Work out the finished part from the listing and answer in its coordinate system (mm). Face numbers are marked on the shaded views. Coordinates: 2 decimals unless noted, no trailing zeros. Order: outer loops, then holes, each group sorted by start corner. A loop starts at its lowest first (then second) coordinate and runs counter-clockwise, first axis right, second up. Notation, with made-up numbers: (17, 45.25) -> (27, 45.25) arc R28 ccw to (27, 79.25) -> close; hole circle Ø1 at (77.25, 37.25). An arc over 180 degrees is marked (long way). Answer as CSV lines item,"result". Start each with the question number.
Item 1: Each of these flat-tipped pins is pushed along its axis until it touches: pin 1 Ø11 at (x, z) = (87.5, -304.5) entering from +Y; pin 2 Ø1 at (x, z) = (195, -235.5) entering from +Y; pin 3 Ø5 at (x, z) = (173, -341.5) entering from +Y. Where does it stop, or does it pass through?
Item 2: For a pull along Z with two mould halves and no side action, classify the marked faces 1 and 2 as pulls with the +Z half, pulls with the -Z half, needs draft (parallel to the pull), parting line crosses it, or undercut.
Item 3: Section A-A (x = 214) is taken. Write down the section's boundary in (y, z), then the cut area to 3 significant figures.
Item 4: Straight lines are drawn through the part: L1, parallel to X at y = 12.25, z = -313; L2, parallel to X at y = 3.25, z = -337.5; L3, parallel to Z at x = 127, y = 2.75. For each, find the intervals that lie inside material, in ascending order.
```python
from build123d import *

# Parameters (mm, degrees)
SKETCH1_W                     = 224.81
SKETCH1_H                     = 138.7
BOTTOM_PLATE_DEPTH            = 4
SKETCH2_W                     = 8
SKETCH2_H                     = 8
SKETCH2_W_2                   = 7
SKETCH2_H_2                   = 7
SIDE_WALLS_DEPTH              = 11
SKETCH11_W                    = 4
SKETCH11_H                    = 123.7
USB_CUTOUT_DEPTH              = 11
CSK_FOR_M3_SFHCS1_D           = 3.2
CSK_FOR_M3_SFHCS1_CSINK_D     = 6.72
CSK_FOR_M3_SFHCS1_CSINK_ANGLE = 90
FILLET1_R                     = 1.5
USB_C_PORT_DEPTH              = 10
SKETCH18_W                    = 15
SKETCH18_H                    = 4.1
BOSS_EXTRUDE1_DEPTH           = 1.5
CHAMFER1_SIZE                 = 2
SKETCH16_R                    = 5
PCB_SUPPORT_DEPTH             = 2
SKETCH17_R                    = 1.5
ALIGNMENT_POSTS_DEPTH         = 2
SKETCH20_R                    = 1.6
PCB_SCREW_CLEARANCE_DEPTH     = 2.15
SKETCH21_W                    = 5.5
SKETCH21_H                    = 5.5
CUT_EXTRUDE2_DEPTH            = 1.8


with BuildPart() as part:
    # Sketch1 → bottom_plate (new body)
    with BuildSketch(Plane(origin=(0, 0, 0), x_dir=(1, 0, 0), z_dir=(0, 1, 0))):
        with Locations((157.396993286, 282.353126042)):
            Rectangle(SKETCH1_W, SKETCH1_H)
    extrude(amount=BOTTOM_PLATE_DEPTH)

    # Sketch2 → side_walls (add)
    with BuildSketch(Plane(origin=(0, 4, 0), x_dir=(1, 0, 0), z_dir=(0, 1, 0))):
        with Locations((48.991993286, 217.003126042)):
            Rectangle(SKETCH2_W, SKETCH2_H)
        with Locations((266.301993286, 216.503126042)):
            Rectangle(SKETCH2_W_2, SKETCH2_H_2)
        with Locations((266.301993286, 348.203126042)):
            Rectangle(SKETCH2_W_2, SKETCH2_H_2)
        with Locations((48.991993286, 348.203126042)):
            Rectangle(SKETCH2_W, SKETCH2_H_2)
    extrude(amount=SIDE_WALLS_DEPTH)

    # Sketch11 → usb_cutout (add)
    with BuildSketch(Plane(origin=(0, 4, 0), x_dir=(1, 0, 0), z_dir=(0, 1, 0))):
        with Locations((46.991993286, 282.853126042)):
            Rectangle(SKETCH11_W, SKETCH11_H)
        Polygon((52.991993286, 213.003126042), (262.801993286, 213.003126042), (262.801993286, 219.003126042), (269.801993286, 219.003126042), (269.801993286, 345.703126042), (262.801993286, 345.703126042), (262.801993286, 351.703126042), (52.991993286, 351.703126042), (52.991993286, 345.703126042), (75.991993286, 345.703126042), (75.991993286, 349.803126042), (90.991993286, 349.803126042), (90.991993286, 345.703126042), (261.801993286, 345.703126042), (261.801993286, 219.003126042), (52.991993286, 219.003126042), align=None)
    extrude(amount=USB_CUTOUT_DEPTH)

    # CSK for M3 SFHCS1 (through all)
    with Locations(Plane(origin=(0, 0, 0), x_dir=(-1, 0, 0), z_dir=(0, -1, 0))):
        with Locations((-48.991993286, 217.003686618), (-265.799879733, 217.003686618), (-265.799879733, 347.703126042), (-48.991993286, 347.703126042)):
            CounterSinkHole(CSK_FOR_M3_SFHCS1_D / 2, CSK_FOR_M3_SFHCS1_CSINK_D / 2, counter_sink_angle=CSK_FOR_M3_SFHCS1_CSINK_ANGLE)

    # Fillet1
    fillet1_edges = [part.edges().sort_by_distance(p)[0] for p in [
        (44.991993286, 7.5, -351.703126042),
        (269.801993286, 7.5, -351.703126042),
        (269.801993286, 7.5, -213.003126042),
        (44.991993286, 7.5, -213.003126042),
    ]]
    fillet(fillet1_edges, radius=FILLET1_R)

    # Sketch14 → usb-c port (cut)
    with BuildSketch(Plane.XY.offset(-349.803126042)):
        with BuildLine():
            Line((80.300245901, 7.7), (86.470717131, 7.7))
            ThreePointArc((86.470717131, 7.7), (87.531377303, 8.139339828), (87.970717131, 9.2))
            Line((87.970717131, 9.2), (87.970717131, 9.590467347))
            ThreePointArc((87.970717131, 9.590467347), (87.531377303, 10.651127519), (86.470717131, 11.090467347))
            Line((86.470717131, 11.090467347), (80.300245901, 11.090467347))
            ThreePointArc((80.300245901, 11.090467347), (79.239585729, 10.651127519), (78.800245901, 9.590467347))
            Line((78.800245901, 9.590467347), (78.800245901, 9.2))
            ThreePointArc((78.800245901, 9.2), (79.239585729, 8.139339828), (80.300245901, 7.7))
        make_face()
    extrude(amount=-USB_C_PORT_DEPTH, mode=Mode.SUBTRACT)

    # Sketch18 → Boss-Extrude1 (add)
    with BuildSketch(Plane(origin=(0, 15, 0), x_dir=(1, 0, 0), z_dir=(0, 1, 0))):
        with Locations((83.491993286, 347.753126042)):
            Rectangle(SKETCH18_W, SKETCH18_H)
    extrude(amount=-BOSS_EXTRUDE1_DEPTH)

    # Chamfer1
    chamfer1_edges = [part.edges().sort_by_distance(p)[0] for p in [
        (83.491993286, 13.5, -349.803126042),
        (83.491993286, 4, -349.803126042),
    ]]
    chamfer(chamfer1_edges, length=CHAMFER1_SIZE)

    # Sketch16 → pcb_support (add)
    with BuildSketch(Plane(origin=(0, 4, 0), x_dir=(1, 0, 0), z_dir=(0, 1, 0))):
        with Locations(Location((55.991993286, 340.003687101, 0), (0, 0, 90))):
            Circle(SKETCH16_R)
        with Locations(Location((56.991993286, 279.503687101, 0), (0, 0, 90))):
            Circle(SKETCH16_R)
        with Locations(Location((132.491993286, 256.003687101, 0), (0, 0, 90))):
            Circle(SKETCH16_R)
        with Locations(Location((253.991993286, 271.003687101, 0), (0, 0, 90))):
            Circle(SKETCH16_R)
        with Locations(Location((254.991993286, 320.503687101, 0), (0, 0, 90))):
            Circle(SKETCH16_R)
        with Locations(Location((156.991993286, 286.503687101, 0), (0, 0, 90))):
            Circle(SKETCH16_R)
        with Locations(Location((171.991993286, 339.003687101, 0), (0, 0, 90))):
            Circle(SKETCH16_R)
        with Locations(Location((127.491993286, 334.503687101, 0), (0, 0, 90))):
            Circle(SKETCH16_R)
        with Locations(Location((173.491993286, 309.003687101, 0), (0, 0, 90))):
            Circle(SKETCH16_R)
        with Locations(Location((198.491993286, 294.003687101, 0), (0, 0, 90))):
            Circle(SKETCH16_R)
        with Locations(Location((180.991993286, 232.503687101, 0), (0, 0, 90))):
            Circle(SKETCH16_R)
        with Locations(Location((84.991993286, 305.503687101, 0), (0, 0, 90))):
            Circle(SKETCH16_R)
        with Locations(Location((156.491993286, 250.253687101, 0), (0, 0, 90))):
            Circle(SKETCH16_R)
        with Locations(Location((132.991993286, 232.503687101, 0), (0, 0, 90))):
            Circle(SKETCH16_R)
    extrude(amount=PCB_SUPPORT_DEPTH)

    # Sketch17 → alignment_posts (add)
    with BuildSketch(Plane(origin=(0, 6, 0), x_dir=(1, 0, 0), z_dir=(0, 1, 0))):
        with Locations(Location((84.991993286, 305.503687101, 0), (0, 0, 270))):
            Circle(SKETCH17_R)
        with Locations(Location((198.491993286, 294.003687101, 0), (0, 0, 270))):
            Circle(SKETCH17_R)
        with Locations(Location((156.491993286, 250.253687101, 0), (0, 0, 270))):
            Circle(SKETCH17_R)
    extrude(amount=ALIGNMENT_POSTS_DEPTH)

    # Sketch20 → pcb screw clearance (cut)
    with BuildSketch(Plane(origin=(0, 6, 0), x_dir=(1, 0, 0), z_dir=(0, 1, 0))):
        with Locations(Location((55.991993286, 340.003687101, 0), (0, 0, 270))):
            Circle(SKETCH20_R)
        with Locations(Location((127.491993286, 334.503687101, 0), (0, 0, 270))):
            Circle(SKETCH20_R)
        with Locations(Location((56.991993286, 279.503687101, 0), (0, 0, 270))):
            Circle(SKETCH20_R)
        with Locations(Location((132.491993286, 256.003687101, 0), (0, 0, 270))):
            Circle(SKETCH20_R)
        with Locations(Location((132.991993286, 232.503687101, 0), (0, 0, 270))):
            Circle(SKETCH20_R)
        with Locations(Location((180.991993286, 232.503687101, 0), (0, 0, 270))):
            Circle(SKETCH20_R)
        with Locations(Location((156.991993286, 286.503687101, 0), (0, 0, 270))):
            Circle(SKETCH20_R)
        with Locations(Location((253.991993286, 271.003687101, 0), (0, 0, 270))):
            Circle(SKETCH20_R)
        with Locations(Location((173.491993286, 309.003687101, 0), (0, 0, 270))):
            Circle(SKETCH20_R)
        with Locations(Location((171.991993286, 339.003687101, 0), (0, 0, 270))):
            Circle(SKETCH20_R)
        with Locations(Location((254.991993286, 320.503687101, 0), (0, 0, 270))):
            Circle(SKETCH20_R)
    extrude(amount=-PCB_SCREW_CLEARANCE_DEPTH, mode=Mode.SUBTRACT)

    # Sketch21 → Cut-Extrude2 (cut)
    with BuildSketch(Plane(origin=(0, 3.85, 0), x_dir=(1, 0, 0), z_dir=(0, 1, 0))):
        with Locations((55.991993286, 340.003687101)):
            Rectangle(SKETCH21_W, SKETCH21_H)
        with Locations((127.491993286, 334.503687101)):
            Rectangle(SKETCH21_W, SKETCH21_H)
        with Locations((56.991993286, 279.503687101)):
            Rectangle(SKETCH21_W, SKETCH21_H)
        with Locations((132.491993286, 256.003687101)):
            Rectangle(SKETCH21_W, SKETCH21_H)
        with Locations((132.991993286, 232.503687101)):
            Rectangle(SKETCH21_W, SKETCH21_H)
        with Locations((180.991993286, 232.503687101)):
            Rectangle(SKETCH21_W, SKETCH21_H)
        with Locations((253.991993286, 271.003687101)):
            Rectangle(SKETCH21_W, SKETCH21_H)
        with Locations((173.491993286, 309.003687101)):
            Rectangle(SKETCH21_W, SKETCH21_H)
        with Locations((171.991993286, 339.003687101)):
            Rectangle(SKETCH21_W, SKETCH21_H)
        with Locations((254.991993286, 320.503687101)):
            Rectangle(SKETCH21_W, SKETCH21_H)
    extrude(amount=-CUT_EXTRUDE2_DEPTH, mode=Mode.SUBTRACT)


solid = part.part
```
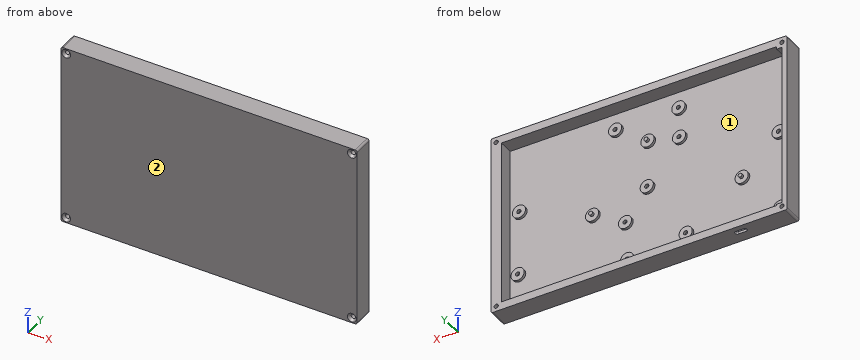
Checked values:
1,pin 1,"stops at y = 8"
1,pin 2,"stops at y = 4"
1,pin 3,"stops at y = 6"
2,face 1,"undercut"
2,face 2,"needs draft"
3,outline,"(0, -351.7) -> (15, -351.7) -> (15, -345.7) -> (4, -345.7) -> (4, -219) -> (15, -219) -> (15, -213) -> (0, -213) -> close"
3,area,"687 mm^2"
4,L1,"x = 44.99 to 48.99, 261.8 to 269.8"
4,L2,"x = 44.99 to 53.24, 58.74 to 169.24, 174.74 to 269.8"
4,L3,"z = -351.7 to -337.25, -331.75 to -213"
